Check sheet for the drawn part. Datum: minimum x, y, z corner. Units: mm. Coordinates: 2 decimals unless noted, no trailing zeros. Write each loop counter-clockwise with the first axis right and the second up, starting at its lowest first coordinate (ties: lowest second). Pieces come first, ordered by that corner, then holes. Notation, with made-up numbers: (-26.75, 0.25) - (-14.75, 0.25) arc R10 ccw to (-14.75, 11.25) - close; hole circle Ø3 at (32.5, -24.5). An arc over 180 degrees is marked (long way). Use one line per item in the form item = value. Start each with the question number.
1. Draft check along Y on the marked faces 1 and 2. Enter one of: +Y half, -Y half, draft (parallel to the pull), parting line (faces both ways), or undercut.
2. Scan lines: line 1 along Y through (x, z) = (27.62, 4.65) (3 decimals); line 2 along X through (y, z) = (34, 1). Record each from-to range of solid material in increasing order.
3. Cross-section at C-C on z = 2.5. Record the boundary of the cut face in (x, y).
4. Cross-section at A-A on x = 35. Record the boundary of the cut face in (y, z), then the cut area to 3 significant figures.
5. Cross-section at D-D on x = 27.62. Record the boundary of the cut face in (y, z) (3 decimals), then the cut area to 3 significant figures.
6. Go/stop test with flat-tipped pins: pin 1 Ø0.8 at (x, y) = (13, 9) entering from +Z; pin 2 Ø1 at (x, y) = (10, 23.5) entering from -Z; pin 3 Ø1 at (x, z) = (13, 5) entering from +Y. Record where each tip stops, or that it passes through.
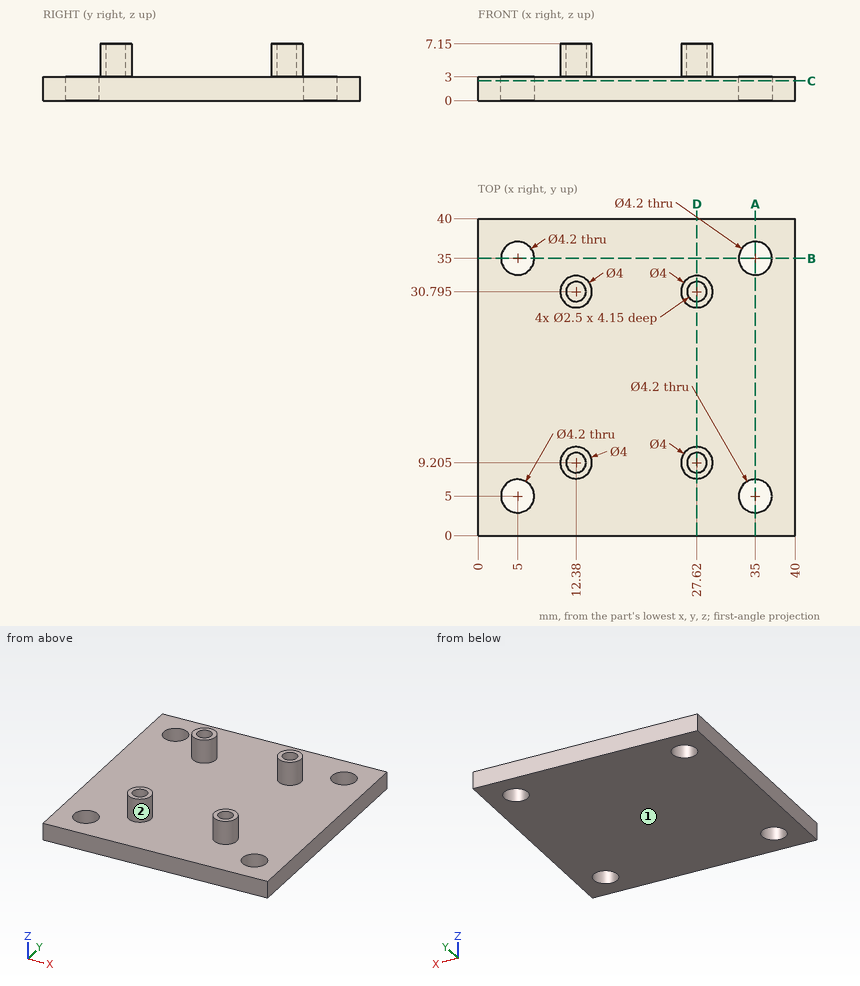
Final values:
q1.face_1 = draft
q1.face_2 = undercut
q2.line_1 = 7.205 to 7.955, 10.455 to 11.205, 28.795 to 29.545, 32.045 to 32.795
q2.line_2 = 0 to 3.15, 6.85 to 33.15, 36.85 to 40
q3.outline = (0, 0) - (40, 0) - (40, 40) - (0, 40) - close; hole circle Ø4.2 at (5, 5); hole circle Ø4.2 at (5, 35); hole circle Ø4.2 at (35, 5); hole circle Ø4.2 at (35, 35)
q4.outline = (0, 0) - (2.9, 0) - (2.9, 3) - (0, 3) - close; (7.1, 0) - (32.9, 0) - (32.9, 3) - (7.1, 3) - close; (37.1, 0) - (40, 0) - (40, 3) - (37.1, 3) - close
q4.area = 94.8 mm²
q5.outline = (0, 0) - (40, 0) - (40, 3) - (32.795, 3) - (32.795, 7.15) - (32.045, 7.15) - (32.045, 3) - (29.545, 3) - (29.545, 7.15) - (28.795, 7.15) - (28.795, 3) - (11.205, 3) - (11.205, 7.15) - (10.455, 7.15) - (10.455, 3) - (7.955, 3) - (7.955, 7.15) - (7.205, 7.15) - (7.205, 3) - (0, 3) - close
q5.area = 132 mm²
q6.pin_1 = 3
q6.pin_2 = 0
q6.pin_3 = 32.79
